Design review of the part built by this model. Coordinates are the model's own, in mm. A direction names the side the tool comes from. Coordinates: 2 decimals unless noted, no trailing zeros. Loops run counter-clockwise (first coordinate to the right, second up) from the corner with the lowest first, then second, coordinate; pieces in that order, holes last. Notation, with made-up numbers: (25, 3.25) - (68, 3.25) arc R13 ccw to (68, 18.25) - close; hole circle Ø3 at (17.25, 14.25). An arc over 180 degrees is marked (long way). One line per question, with ' | ' between items.
from build123d import *

# Parameters (mm, degrees)
SKETCH1_R           = 5
BOSS_EXTRUDE1_DEPTH = 16.5
SKETCH2_R           = 7.5
BOSS_EXTRUDE2_DEPTH = 39.5
SKETCH16_W          = 3
SKETCH16_H          = 64.5
CHAMFER_1_SIZE      = 2.5
SKETCH9_R           = 5
EXTRUDE_1_DEPTH     = 20
EXTRUDE_1_TAPER     = 2.8625
SKETCH_1_R          = 3.999966835
EXTRUDE_2_DEPTH     = 7.5
CHAMFER_2_SIZE      = 1
CUT_EXTRUDE_1_DEPTH = 10


with BuildPart() as part:
    # Sketch1 → Boss-Extrude1 (new body)
    with BuildSketch(Plane.XY):
        Circle(SKETCH1_R)
    extrude(amount=BOSS_EXTRUDE1_DEPTH)

    # Sketch2 → Boss-Extrude2 (add)
    with BuildSketch(Plane.XY.offset(16.5)):
        Circle(SKETCH2_R)
    extrude(amount=BOSS_EXTRUDE2_DEPTH)

    # Sketch16 → Cut-Revolve1 (revolve, cut)
    with BuildSketch(Plane(origin=(0, 0, 0), x_dir=(1, 0, 0), z_dir=(0, 1, 0)), mode=Mode.PRIVATE) as cut_revolve1_sk:
        with Locations((6.5, -51.25)):
            Rectangle(SKETCH16_W, SKETCH16_H)
    revolve(cut_revolve1_sk.sketch.rotate(Axis((0, 0, 56), (0, 0, -1)), 180), axis=Axis((0, 0, 56), (0, 0, -1)), mode=Mode.SUBTRACT)

    # Фаска1
    chamfer_1_edges = [part.edges().sort_by_distance(p)[0] for p in [
        (-5, 0, 16.5),
    ]]
    chamfer(chamfer_1_edges, length=CHAMFER_1_SIZE - 0.0001)  # a hair under: the kernel refuses the full size

    # Sketch9 → Бобышка-Вытянуть1 (add)
    with BuildSketch(Plane(origin=(0, 0, 0), x_dir=(-1, 0, 0), z_dir=(0, 0, -1))):
        Circle(SKETCH9_R)
    extrude(amount=EXTRUDE_1_DEPTH, taper=EXTRUDE_1_TAPER)

    # Эскиз1 → Бобышка-Вытянуть2 (add)
    with BuildSketch(Plane(origin=(0, 0, -20), x_dir=(-1, 0, 0), z_dir=(0, 0, -1))):
        Circle(SKETCH_1_R)
    extrude(amount=EXTRUDE_2_DEPTH)

    # Фаска2
    chamfer_2_edges = [part.edges().sort_by_distance(p)[0] for p in [
        (5, 0, 56),
        (3.999966835, 0, -27.5),
    ]]
    chamfer(chamfer_2_edges, length=CHAMFER_2_SIZE)

    # Sketch38 → Вырез-Вытянуть1 (cut)
    with BuildSketch(Plane(origin=(0, 0, 0), x_dir=(1, 0, 0), z_dir=(0, 1, 0))):
        with BuildLine():
            Line((-1.5, -3), (-1.5, -67.243921767))
            ThreePointArc((-1.5, -67.243921767), (0, -68.743921767), (1.5, -67.243921767))
            Line((1.5, -67.243921767), (1.5, -3))
            ThreePointArc((1.5, -3), (0, -1.5), (-1.5, -3))
        make_face()
    extrude(amount=CUT_EXTRUDE_1_DEPTH, mode=Mode.SUBTRACT)


solid = part.part
Q1. Take a section at A-A (z = -21). Give the boundary of the cut face in (x, y), plus the area to 3 significant figures.
Returned:
outline: circle Ø8 at (0, 0) | area: 50.3 mm²
Q2. Take a section at B-B (z = 40). Give the boundary of the cut face in (x, y), plus the area to 3 significant figures.
Returned:
outline: (-1.5, 0) - (-1.5, 4.77) arc R5 ccw (long way) to (1.5, 4.77) - (1.5, 0) - close | area: 63.8 mm²
Q3. Take a section at C-C (z = -12). Give the boundary of the cut face in (x, y).
Returned:
outline: circle Ø8.8 at (0, 0)
Q4. For pin 1 (1 mm diameter, centred on x = 5, z = 6, fed in from -Y); pin 2 (8 mm diameter, centred on y = 3.5, z = 29, fed in from -X); pin 3 (2.5 mm diameter, centred on x = -0.5, z = 27, fed in from +Y), all flat-tipped, find the tip position at first contact; note any pin that passes through.
Returned:
pin 1: stops at y = -2.18 | pin 2: stops at x = -5 | pin 3: stops at y = 4.77
Q5. To check wall thickness, follow line 1 along X through (y, z) = (1.25, 24); line 2 along Y through (x, z) = (3, 37.5); line 3 along X through (y, z) = (2.5, 50.5). State the ranges of each line that lie inside material, in increasing order.
Returned:
line 1: x = -4.84 to -1.5, 1.5 to 4.84 | line 2: y = -4 to 4 | line 3: x = -4.33 to -1.5, 1.5 to 4.33
Q6. Draft analysis for pull direction X (two halves, no side actions). For faces 5 (the flat face through (0, 0, 28)), 6 (the flat face through (0, 0, -27.5)), 7 (the conical face through (0.165, -4.156, 55.84)), state which applies: +X half, -X half, draft (parallel to the pull), parting line (faces both ways), or undercut.
Returned:
face 5: undercut | face 6: draft | face 7: parting line
Q7. Tool access review of faces 1 (the cylindrical face through (0, -5, 37)), 2 (the cylindrical face through (-1.08, -4.88, 6.9)), 3 (the cylindrical face through (-0.309, -7.494, 17.732)), 4 (the cylindrical face through (0, 2.5, 1.5)): name each direction out of +Z, -Z, +X, -X, +Y, -Y from which nothing blocks a thin tool from reaching the whole face with its end or side.
Returned:
face 1: +Z | face 2: -Z | face 3: +Z, -Z | face 4: +Z, +Y
